Check sheet for the drawn part. Datum: minimum x, y, z corner. Units: mm. A direction names the side the tool comes from. Give positions to 0.01 mm unless a question says otherwise; leave off trailing zeros. Write each loop counter-clockwise with the first axis right and the second up, starting at its lowest first coordinate (ties: lowest second). Pieces come first, ordered by that corner, then holes. Notation, with made-up numbers: (-24, 10.25) -> (-20, 10.25) arc R26 cw to (-20, 25.25) -> close; hole circle Ø10 at (-34.75, 27). An arc over 180 degrees is marked (long way). Write item = value, one per line. Start each with the question number.
1. Thickness scan on line 1 along Y through (x, z) = (15, 9.75); line 2 along Z through (x, y) = (40.5, 48). Record the ranges inside material, lowest first.
2. Depth check by flat-ended pin: P1, Ø6, axis at y = 34.5, z = 9.5, coming from the +X side; P2, Ø1.2, axis at y = 33.5, z = 7.5, coming from the -X side; P3, Ø12, axis at x = 39.5, y = 30, coming from the +Z side. Enter the tip coordinate at first touch or a pass-through.
3. Set-up check for the marked faces 1 and 2: record each of +Z, -Z, +X, -X, +Y, -Y from which the full face is reachable in a straight line by a thin tool's end or side.
4. Cross-section at C-C, the plane x = 61. Record the cut outline in (y, z).
5. Cross-section at D-D, the plane y = 43. Record the cut outline in (x, z).
6. Cross-section at A-A, the plane y = 21. Record the cut outline in (x, z).
7. Cross-section at B-B, the plane z = 6.25. Record the cut outline in (x, y).
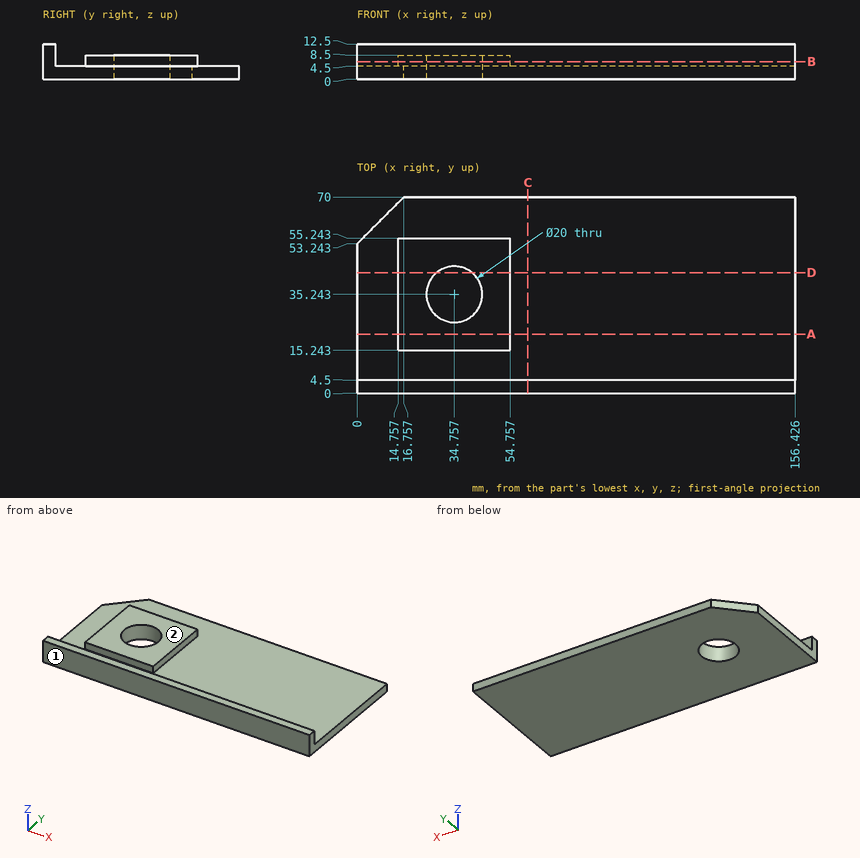
Answers:
q1.line_1 = 0 to 4.5
q1.line_2 = 0 to 8.5
q2.P1 = 54.76
q2.P2 = 14.76
q2.P3 = 8.5
q3.face_1 = +Z, -Z, +X, -X, -Y
q3.face_2 = +Z, +X, -X, +Y
q4.outline = (0, 0) -> (70, 0) -> (70, 4.5) -> (4.5, 4.5) -> (4.5, 12.5) -> (0, 12.5) -> close
q5.outline = (0, 0) -> (28.45, 0) -> (28.45, 8.5) -> (14.76, 8.5) -> (14.76, 4.5) -> (0, 4.5) -> close; (41.07, 0) -> (156.43, 0) -> (156.43, 4.5) -> (54.76, 4.5) -> (54.76, 8.5) -> (41.07, 8.5) -> close
q6.outline = (0, 0) -> (156.43, 0) -> (156.43, 4.5) -> (54.76, 4.5) -> (54.76, 8.5) -> (14.76, 8.5) -> (14.76, 4.5) -> (0, 4.5) -> close
q7.outline = (0, 0) -> (156.43, 0) -> (156.43, 4.5) -> (0, 4.5) -> close; (14.76, 15.24) -> (54.76, 15.24) -> (54.76, 55.24) -> (14.76, 55.24) -> close; hole circle Ø20 at (34.76, 35.24)
